The listing builds one solid part. Answer for the finished solid, in the listing's coordinates (mm). A direction names the side the tool comes from. Coordinates: 2 decimals unless noted, no trailing zeros. Loops run counter-clockwise (first coordinate to the right, second up) from the corner with the lowest first, then second, coordinate; pieces in that order, holes last. Notation, with made-up numbers: M 36.25,45 L 84.25,45 A34 ccw 84.25,84 Z; hole C -1.5,38.25 d7. An arc over 180 degrees is marked long. Return JSON: item names as keys, results as strings. Group by question number.
1. Straight lines are drawn through the part: L1, parallel to Z at x = 790.5, y = 186; L2, parallel to Y at x = 191, z = 1896. For each, find the intervals that lie inside material, in ascending order. Write a range as from..to.
2. Section A-A (x = 217) is taken. Write down the section's boundary in (y, z).
3. Given P1, Ø8, axis at y = 502, z = 1490, coming from the -X side; P2, Ø1.5, axis at x = 560.5, z = 1374, coming from the -Y side; P3, Ø6, axis at x = 397, z = 1361.5, coming from the +Y side, each flat-ended and moving along its own axis, determine where each tip first touches the part or whether it passes through.
4. The mould has two halves that part along X. Classify faces 1 (the face through (419, 330, 2000)), 2 (the face through (100, 379, 1013)), 3 (the face through (189.05, -9.86, 141.33)): pulls with the +X half, pulls with the -X half, needs draft (parallel to the pull), parting line crosses it, or undercut.
5. Section D-D (z = 1634) is taken. Write down the section's boundary in (x, y).
6. Section B-B (y = 590.5) is taken. Write down the section's boundary in (x, z), then the cut area to 3 significant figures.
7. Which of the six approach directions +Z, -Z, +X, -X, +Y, -Y give full straight-line access (tool end or side, diameter ignored) to faces 4 (the face through (470, 379, 100)), 5 (the face through (739.05, -9.86, 141.33)), 6 (the face through (149, -20, 149))?
8. Section C-C (z = 150) is taken. Write down the section's boundary in (x, y).
```python
from build123d import *

# Parameters (mm, degrees)
BOSS_EXTRUDE1_DEPTH = 2000
SKETCH2_W           = 1015.39839311
SKETCH2_H           = 1800
CUT_EXTRUDE1_DEPTH  = 550
SKETCH3_R           = 40
BOSS_EXTRUDE2_DEPTH = 20


with BuildPart() as part:
    # Sketch1 → Boss-Extrude1 (new body)
    with BuildSketch(Plane.XY):
        with BuildLine():
            Line((0, 0), (850, 0))
            Line((850, 0), (850, 630))
            ThreePointArc((850, 630), (844.142135624, 644.142135624), (830, 650))
            Line((830, 650), (0, 650))
            Line((0, 650), (0, 0))
        make_face()
    extrude(amount=BOSS_EXTRUDE1_DEPTH)

    # Sketch2 → Cut-Extrude1 (cut)
    with BuildSketch(Plane(origin=(0, 650, 0), x_dir=(1, 0, 0), z_dir=(0, 1, 0))):
        with Locations((607.699196555, -1000)):
            Rectangle(SKETCH2_W, SKETCH2_H)
    extrude(amount=-CUT_EXTRUDE1_DEPTH, mode=Mode.SUBTRACT)

    # Sketch3 → Boss-Extrude2 (add)
    with BuildSketch(Plane.XZ):
        with Locations(Location((150, 1850, 0), (0, 0, 90))):
            Circle(SKETCH3_R)
        with Locations(Location((700, 1850, 0), (0, 0, 90))):
            Circle(SKETCH3_R)
        with Locations(Location((700, 150, 0), (0, 0, 90))):
            Circle(SKETCH3_R)
        with Locations(Location((150, 150, 0), (0, 0, 90))):
            Circle(SKETCH3_R)
    extrude(amount=BOSS_EXTRUDE2_DEPTH)


solid = part.part
```
Worked out:
{
 "1": {"L1": "0..100, 1900..2000", "L2": "0..100"},
 "2": {"outline": "M 0,0 L 650,0 L 650,100 L 100,100 L 100,1900 L 650,1900 L 650,2000 L 0,2000 Z"},
 "3": {"P1": "x = 0", "P2": "y = 0", "P3": "y = 100"},
 "4": {"face 1": "needs draft", "face 2": "pulls with the +X half", "face 3": "undercut"},
 "5": {"outline": "M 0,0 L 850,0 L 850,100 L 100,100 L 100,650 L 0,650 Z"},
 "6": {"outline": "M 0,0 L 850,0 L 850,100 L 100,100 L 100,1900 L 850,1900 L 850,2000 L 0,2000 Z", "area": "350,000 mm^2"},
 "7": {"face 4": "+X, +Y", "face 5": "-Y", "face 6": "+Z, -Z, +X, -X, -Y"},
 "8": {"outline": "M 0,0 L 110,0 L 110,-20 L 190,-20 L 190,0 L 660,0 L 660,-20 L 740,-20 L 740,0 L 850,0 L 850,100 L 100,100 L 100,650 L 0,650 Z"}
}
